Here's the drawing with two shaded views (mm, measured from the low corner). I have some questions. A direction names the side the tool comes from. Round coordinates to 2 decimals unless told otherwise and drop trailing zeros. Loops run counter-clockwise (first coordinate to the right, second up) from the corner with the lowest first, then second, coordinate; pieces in that order, holes last. Notation, with made-up numbers: M -2.75,-35 L 10.25,-35 A22 ccw 10.25,4 Z; hole C -17.5,87.5 d1. An arc over 180 degrees is marked long. One line per item, written item: value. Start each with the question number.
Q1. Thinking about a two-plate mould opening in Y: for the marked faces 3, 4 and 5, which applies, released by +Y, released by -Y, zero draft, split by the parting line, or undercut?
Q2. I'm going to push flat-ended pins straight in: pin 1 Ø9.5 at (x, y) = (65.09, 38.1) entering from +Z; pin 2 Ø6.5 at (x, y) = (38.1, 11.11) entering from -Z; pin 3 Ø3 at (x, z) = (41.5, 26.5) entering from -Y; pin 4 Ø23 at (x, y) = (27.5, 23) entering from +Z. Where does each tip first touch, or does it pass through?
Q3. Imagine slicing it at C-C (z = 41). Please give me the cut outline in (x, y) (1 decimal), then the cut area to 3 significant figures.
Q4. Imagine slicing it at A-A (y = 26). Please give me the cut outline in (x, z).
Q5. Which directions (+Z, -Z, +X, -X, +Y, -Y) give clear straight access to the entire face, cutting with the end or side of a thin tool? Please do the marked faces 1 and 2.
Q6. Please list where these lines run through material, in increasing order: line 1 along Y through (x, z) = (38.1, 0.7); line 2 along Z through (x, y) = (27, 40); line 3 along Z through (x, y) = (69.5, 25.5).
Q7. Imagine slicing it at B-B (x = 38.1). Give the number of separate pieces and of enclosed holes in the cut face, then the cut area to 3 significant figures.
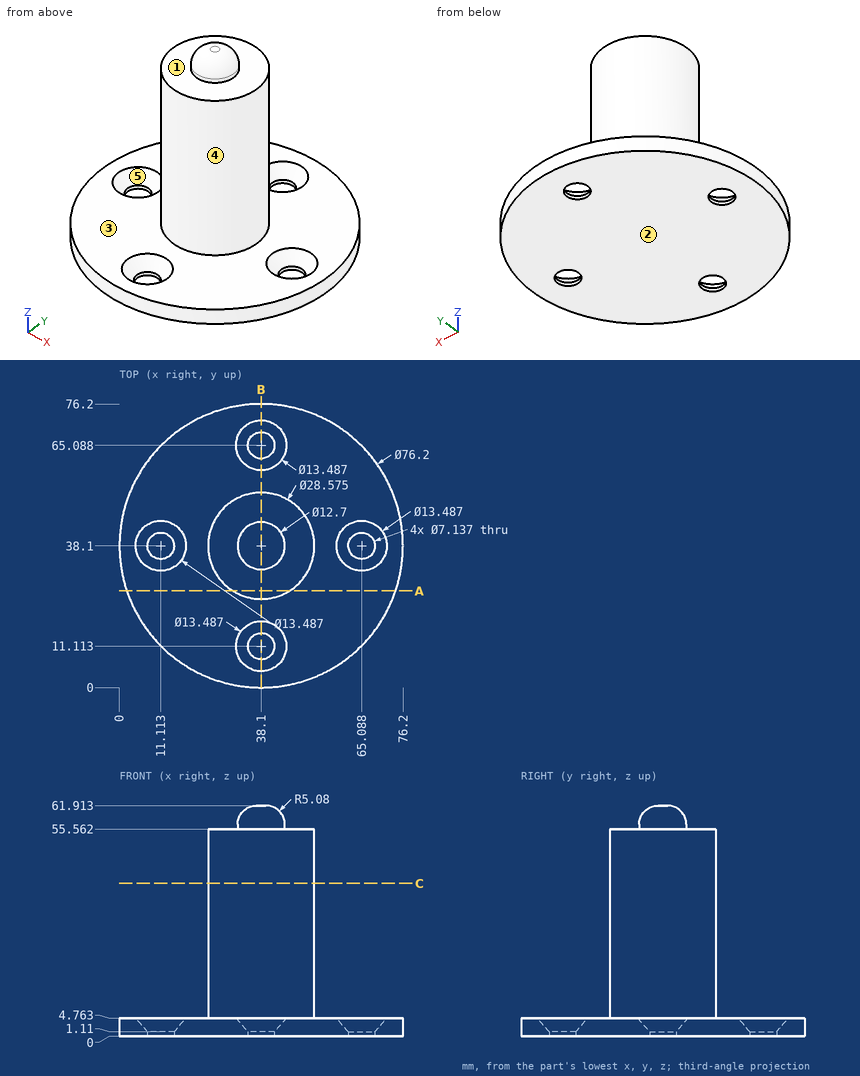
Report:
1. face 3: zero draft
1. face 4: split by the parting line
1. face 5: undercut
2. pin 1: stops at z = 2.47
2. pin 2: passes through
2. pin 3: stops at y = 23.94
2. pin 4: stops at z = 55.56
3. outline: C 38.1,38.1 d28.6
3. area: 641 mm²
4. outline: M 1.97,0 L 74.23,0 L 74.23,4.76 L 45.7,4.76 L 45.7,55.56 L 30.5,55.56 L 30.5,4.76 L 1.97,4.76 Z
5. face 1: +Z
5. face 2: -Z, +X, -X, +Y, -Y
6. line 1: y = 0 to 7.54, 14.68 to 61.52, 68.66 to 76.2
6. line 2: z = 0 to 55.56
6. line 3: z = 0 to 4.76
7. separate pieces: 3
7. enclosed holes: 0
7. area: 1,790 mm²
